Design review of the part built by this model. Coordinates are the model's own, in mm. Coordinates: 2 decimals unless noted, no trailing zeros. Order: outer loops, then holes, each group sorted by start corner. A loop starts at its lowest first (then second) coordinate and runs counter-clockwise, first axis right, second up. Notation, with made-up numbers: (-32.75, -9.5) - (22.25, -9.5) arc R17 cw to (22.25, 15.5) - close; hole circle Ø4 at (48, -13). An arc over 180 degrees is marked (long way). Write item = value, one per line. Start each with the question number.
```python
from build123d import *

# Parameters (mm, degrees)
RESSALTO_EXTRUS_O1_DEPTH = 0.2
RESSALTO_EXTRUS_O2_DEPTH = 0.2
CORTE_EXTRUS_O1_DEPTH    = 1
FILETE1_R                = 0.05
RESSALTO_EXTRUS_O3_DEPTH = 0.145
PADR_O_LINEAR1_COUNT     = 2
PADR_O_LINEAR1_PITCH     = 0.505
CORTE_EXTRUS_O2_DEPTH    = 0.3


with BuildPart() as part:
    # Esboço1 → Ressalto-extrusão1 (new body)
    with BuildSketch(Plane.XY):
        with BuildLine():
            Line((76.710328142, 206.616112347), (76.710328142, 206.416112347))
            Line((76.710328142, 206.416112347), (76.657349848, 206.416112347))
            Line((76.657349848, 206.416112347), (76.657349848, 206.116112347))
            Line((76.657349848, 206.116112347), (76.645328142, 206.116112347))
            Line((76.645328142, 206.116112347), (76.610328142, 206.116112347))
            Line((76.610328142, 206.116112347), (76.560328142, 206.116112347))
            ThreePointArc((76.560328142, 206.116112347), (76.524972803, 206.101467686), (76.510328142, 206.066112347))
            Line((76.510328142, 206.066112347), (76.510328142, 205.966112347))
            Line((76.510328142, 205.966112347), (76.110328142, 205.966112347))
            Line((76.110328142, 205.966112347), (76.081970009, 205.966112347))
            Line((76.081970009, 205.966112347), (75.910328142, 205.966112347))
            Line((75.910328142, 205.966112347), (75.595453106, 206.080717488))
            ThreePointArc((75.595453106, 206.080717488), (75.537376388, 206.073071543), (75.510328142, 206.021112347))
            Line((75.510328142, 206.021112347), (75.510328142, 205.971112347))
            Line((75.510328142, 205.971112347), (75.410328142, 205.971112347))
            Line((75.410328142, 205.971112347), (75.309933917, 206.02907498))
            ThreePointArc((75.309933917, 206.02907498), (75.273690046, 206.034493063), (75.243486264, 206.013739619))
            ThreePointArc((75.243486264, 206.013739619), (75.229104336, 206.000793024), (75.210328142, 205.996112347))
            Line((75.210328142, 205.996112347), (75.160328142, 205.996112347))
            Line((75.160328142, 205.996112347), (74.960328142, 206.041112347))
            Line((74.960328142, 206.041112347), (70.860328142, 206.041112347))
            Line((70.860328142, 206.041112347), (70.560328142, 206.141112347))
            Line((70.560328142, 206.141112347), (70.560328142, 206.391112347))
            Line((70.560328142, 206.391112347), (70.860328142, 206.491112347))
            Line((70.860328142, 206.491112347), (74.960328142, 206.491112347))
            Line((74.960328142, 206.491112347), (75.150344741, 206.536112347))
            Line((75.150344741, 206.536112347), (75.210328142, 206.536112347))
            ThreePointArc((75.210328142, 206.536112347), (75.229104336, 206.53143167), (75.243486264, 206.518485075))
            ThreePointArc((75.243486264, 206.518485075), (75.273690046, 206.497731631), (75.309933917, 206.503149714))
            Line((75.309933917, 206.503149714), (75.410328142, 206.561112347))
            Line((75.410328142, 206.561112347), (75.510328142, 206.561112347))
            Line((75.510328142, 206.561112347), (75.510328142, 206.511112347))
            ThreePointArc((75.510328142, 206.511112347), (75.540942979, 206.456830135), (75.60323487, 206.454946752))
            Line((75.60323487, 206.454946752), (75.910328142, 206.616112347))
            Line((75.910328142, 206.616112347), (76.081970009, 206.616112347))
            Line((76.081970009, 206.616112347), (76.110328142, 206.616112347))
            Line((76.110328142, 206.616112347), (76.710328142, 206.616112347))
        make_face()
    extrude(amount=RESSALTO_EXTRUS_O1_DEPTH)

    # Esboço2 → Ressalto-extrusão2 (add)
    with BuildSketch(Plane.XZ.offset(-206.416112347)):
        with BuildLine():
            Line((76.710328142, 0), (76.710328142, 0.2))
            ThreePointArc((76.710328142, 0.2), (76.851749499, 0.258578644), (76.910328142, 0.4))
            Line((76.910328142, 0.4), (76.910328142, 2.68))
            ThreePointArc((76.910328142, 2.68), (77.02748543, 2.962842712), (77.310328142, 3.08))
            Line((77.310328142, 3.08), (78.110328142, 3.08))
            Line((78.110328142, 3.08), (78.110328142, 2.88))
            Line((78.110328142, 2.88), (77.310328142, 2.88))
            ThreePointArc((77.310328142, 2.88), (77.168906786, 2.821421356), (77.110328142, 2.68))
            Line((77.110328142, 2.68), (77.110328142, 0.4))
            ThreePointArc((77.110328142, 0.4), (76.993170855, 0.117157288), (76.710328142, 0))
        make_face()
    extrude(amount=-RESSALTO_EXTRUS_O2_DEPTH)

    # Esboço3 → Corte-extrusão1 (cut)
    with BuildSketch(Plane(origin=(0, 206.491112347, 0), x_dir=(1, 0, 0), z_dir=(0, 1, 0))):
        Polygon((70.560328142, -0.1), (70.475949981, -0.1), (70.475949981, -0.288700335), (70.860328142, -0.288700335), (70.860328142, -0.2), align=None)
    extrude(amount=-CORTE_EXTRUS_O1_DEPTH, mode=Mode.SUBTRACT)

    # Filete1
    filete1_edges = [part.edges().sort_by_distance(p)[0] for p in [
        (78.110328142, 206.616112347, 2.98),
        (78.110328142, 206.416112347, 2.98),
    ]]
    fillet(filete1_edges, radius=FILETE1_R)

    # Esboço4 → Ressalto-extrusão3 (add)
    with BuildSketch(Plane(origin=(0, 206.616112347, 0), x_dir=(1, 0, 0), z_dir=(0, 1, 0))):
        Polygon((76.057628142, -0.2), (76.310328142, -0.2624), (76.310328142, -0.2), align=None)
    ressalto_extrus_o3 = extrude(amount=-RESSALTO_EXTRUS_O3_DEPTH)

    # Padrão linear1: Ressalto-extrusão3 ×2
    with Locations(*[(0, -i * PADR_O_LINEAR1_PITCH, 0) for i in range(1, PADR_O_LINEAR1_COUNT)]):
        add(ressalto_extrus_o3)

    # Esboço5 → Corte-extrusão2 (cut)
    with BuildSketch(Plane.XZ.offset(-206.116112347)):
        Polygon((76.657349848, 0.16), (76.645349848, 0.16), (76.608838995, 0.2), (76.608838995, 0.232444762), (76.679680574, 0.232444762), (76.679680574, 0.16), align=None)
        Polygon((76.608838995, 0), (76.645349848, 0.04), (76.679680574, 0.04), (76.679680574, -0.014078239), (76.608838995, -0.014078239), align=None)
    extrude(amount=-CORTE_EXTRUS_O2_DEPTH, mode=Mode.SUBTRACT)


solid = part.part
```
Item 1: Add section C-C on x = 77.75. Give the boundary of the cut face in (y, z).
Item 2: For P1, Ø1.5, axis at x = 74.5, z = 1.5, coming from the -Y side; P2, Ø1.2, axis at x = 77.5, z = 1.5, coming from the -Y side, all flat-tipped, find the tip position at first contact; note any pin that passes through.
Item 3: For line 1 (Z direction, x = 74.25, y = 206.1); line 2 (X direction, y = 206.45, z = 2); line 3 (Y direction, x = 77, z = 0.7), list the stretches that pass through material, from the lowest coordinate up.
Item 4: Add section B-B on z = 2.05. Give the boundary of the cut face in (x, y), plus the area to 3 significant figures.
Worked out:
q1.outline = (206.42, 2.88) - (206.62, 2.88) - (206.62, 3.08) - (206.42, 3.08) - close
q2.P1 = through
q2.P2 = 206.42
q3.line_1 = 0 to 0.2
q3.line_2 = 76.91 to 77.11
q3.line_3 = 206.42 to 206.62
q4.outline = (76.91, 206.42) - (77.11, 206.42) - (77.11, 206.62) - (76.91, 206.62) - close
q4.area = 0.0400 mm2
